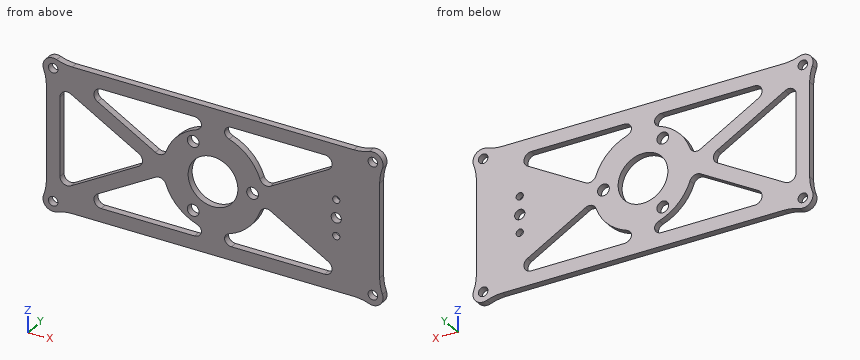
from build123d import *

# Parameters (mm, degrees)
SKETCH_1_R          = 2.1
EXTRUDE_1_DEPTH     = 3
SKETCH_1_R_2        = 22
SKETCH_1_R_3        = 2.6
SKETCH_1_R_4        = 11
EXTRUDE_1_2_DEPTH   = 3
EXTRUDE_START       = -3
EXTRUDE_2_DEPTH     = 3
FILLET_1_R          = 3.2
FILLET_2_R          = 20
EXTRUDE_4_DEPTH     = 3
SKETCH_4_R          = 2.25
SKETCH_4_R_2        = 1.6
CUT_EXTRUDE_1_DEPTH = 83.47010732


with BuildPart() as part:
    # Sketch 1 → Extrude 1 (new body)
    with BuildSketch(Plane(origin=(0, 0, 0), x_dir=(1, 0, 0), z_dir=(0, 1, 0))):
        with BuildLine():
            Line((-67.322682271, -32.275282576), (67.322682271, -32.275282576))
            ThreePointArc((67.322682271, -32.275282576), (73.858764752, -32.457263091), (73.676784237, -25.92118061))
            Line((73.676784237, -25.92118061), (73.676784237, 25.92118061))
            ThreePointArc((73.676784237, 25.92118061), (73.858764752, 32.457263091), (67.322682271, 32.275282576))
            Line((67.322682271, 32.275282576), (-67.322682271, 32.275282576))
            ThreePointArc((-67.322682271, 32.275282576), (-73.858764752, 32.457263091), (-73.676784237, 25.92118061))
            Line((-73.676784237, 25.92118061), (-73.676784237, -25.92118061))
            ThreePointArc((-73.676784237, -25.92118061), (-73.858764752, -32.457263091), (-67.322682271, -32.275282576))
        make_face()
        with Locations(Location((70.676784237, -29.275282576, 0), (0, 0, 270))):
            Circle(SKETCH_1_R, mode=Mode.SUBTRACT)
        with Locations(Location((-70.676784237, -29.275282576, 0), (0, 0, 270))):
            Circle(SKETCH_1_R, mode=Mode.SUBTRACT)
        with Locations(Location((70.676784237, 29.275282576, 0), (0, 0, 270))):
            Circle(SKETCH_1_R, mode=Mode.SUBTRACT)
        with Locations(Location((-70.676784237, 29.275282576, 0), (0, 0, 270))):
            Circle(SKETCH_1_R, mode=Mode.SUBTRACT)
        with BuildLine():
            Line((-67.322682271, 26.275282576), (67.322682271, 26.275282576))
            ThreePointArc((67.322682271, 26.275282576), (67.494803722, 26.093302061), (67.676784237, 25.92118061))
            Line((67.676784237, 25.92118061), (67.676784237, -25.92118061))
            ThreePointArc((67.676784237, -25.92118061), (67.494803722, -26.093302061), (67.322682271, -26.275282576))
            Line((67.322682271, -26.275282576), (-67.322682271, -26.275282576))
            ThreePointArc((-67.322682271, -26.275282576), (-67.494803722, -26.093302061), (-67.676784237, -25.92118061))
            Line((-67.676784237, -25.92118061), (-67.676784237, 25.92118061))
            ThreePointArc((-67.676784237, 25.92118061), (-67.494803722, 26.093302061), (-67.322682271, 26.275282576))
        make_face(mode=Mode.SUBTRACT)
    extrude(amount=EXTRUDE_1_DEPTH)



with BuildPart() as body_2:
    # Sketch 1 → Extrude 1 2 (new body)
    with BuildSketch(Plane(origin=(0, 0, 0), x_dir=(1, 0, 0), z_dir=(0, 1, 0))):
        with Locations(Location((0, 0, 0), (0, 0, 270))):
            Circle(SKETCH_1_R_2)
        with Locations(Location((-8.75, 15.155444566, 0), (0, 0, 270))):
            Circle(SKETCH_1_R_3, mode=Mode.SUBTRACT)
        with Locations(Location((0, 0, 0), (0, 0, 270))):
            Circle(SKETCH_1_R_4, mode=Mode.SUBTRACT)
        with Locations(Location((-8.75, -15.155444566, 0), (0, 0, 270))):
            Circle(SKETCH_1_R_3, mode=Mode.SUBTRACT)
        with Locations(Location((17.5, 0, 0), (0, 0, 270))):
            Circle(SKETCH_1_R_3, mode=Mode.SUBTRACT)
    extrude(amount=EXTRUDE_1_2_DEPTH)


with BuildPart() as part_1:
    add(part.part)

    add(body_2.part)  # Extrude 2 merges body 2
    # Sketch 2 → Extrude 2 (add)
    with BuildSketch(Plane(origin=(0, 3, 0), x_dir=(1, 0, 0), z_dir=(0, 1, 0)).offset(EXTRUDE_START)):
        with BuildLine():
            Line((-5, 26.275282576), (-5, 21.424285286))
            ThreePointArc((-5, 21.424285286), (0, 22), (5, 21.424285286))
            Line((5, 21.424285286), (5, 26.275282576))
            Line((5, 26.275282576), (-5, 26.275282576))
        make_face()
        with BuildLine():
            Line((5, -26.275282576), (5, -21.424285286))
            ThreePointArc((5, -21.424285286), (0, -22), (-5, -21.424285286))
            Line((-5, -21.424285286), (-5, -26.275282576))
            Line((-5, -26.275282576), (5, -26.275282576))
        make_face()
        with BuildLine():
            Line((-67.676784237, 23.012880146), (-27.981475463, 0))
            Line((-27.981475463, 0), (-67.676784237, -23.012880146))
            Line((-67.676784237, -23.012880146), (-67.676784237, -25.92118061))
            ThreePointArc((-67.676784237, -25.92118061), (-67.494803722, -26.093302061), (-67.322682271, -26.275282576))
            Line((-67.322682271, -26.275282576), (-61.341206808, -26.275282576))
            Line((-61.341206808, -26.275282576), (-21.747820556, -3.321490792))
            ThreePointArc((-21.747820556, -3.321490792), (-22, 0), (-21.747820556, 3.321490792))
            Line((-21.747820556, 3.321490792), (-61.341206808, 26.275282576))
            Line((-61.341206808, 26.275282576), (-67.322682271, 26.275282576))
            ThreePointArc((-67.322682271, 26.275282576), (-67.494803722, 26.093302061), (-67.676784237, 25.92118061))
            Line((-67.676784237, 25.92118061), (-67.676784237, 23.012880146))
        make_face()
        with BuildLine():
            Line((61.341206808, 26.275282576), (21.747820556, 3.321490792))
            ThreePointArc((21.747820556, 3.321490792), (22, 0), (21.747820556, -3.321490792))
            Line((21.747820556, -3.321490792), (61.341206808, -26.275282576))
            Line((61.341206808, -26.275282576), (67.322682271, -26.275282576))
            ThreePointArc((67.322682271, -26.275282576), (67.494803722, -26.093302061), (67.676784237, -25.92118061))
            Line((67.676784237, -25.92118061), (67.676784237, -23.012880146))
            Line((67.676784237, -23.012880146), (27.981475463, 0))
            Line((27.981475463, 0), (67.676784237, 23.012880146))
            Line((67.676784237, 23.012880146), (67.676784237, 25.92118061))
            ThreePointArc((67.676784237, 25.92118061), (67.494803722, 26.093302061), (67.322682271, 26.275282576))
            Line((67.322682271, 26.275282576), (61.341206808, 26.275282576))
        make_face()
    extrude(amount=EXTRUDE_2_DEPTH)

    # Fillet 1
    # the kernel refuses this fillet: 3.2 mm, written as the material it adds along each edge
    with BuildSketch(Plane(origin=(-27.981475463, 0, 0), x_dir=(-0.8651295335829952, 0, -0.5015484922940843), z_dir=(0, 1, 0))) as fillet_1_piece_1:
        with BuildLine():
            CenterArc((FILLET_1_R * 1.72491702572, FILLET_1_R), FILLET_1_R, 150.205000829, 119.794999171)
            Line((FILLET_1_R * 0.857108199306, FILLET_1_R * 1.49689821976), (0, 0))
            Line((0, 0), (FILLET_1_R * 1.72491702572, 0))
        make_face()
    extrude(amount=3)
    with BuildSketch(Plane(origin=(-67.676784237, 0, 23.012880146), x_dir=(0, 0, -1), z_dir=(0, 1, 0))) as fillet_1_piece_2:
        with BuildLine():
            CenterArc((FILLET_1_R * 1.73563429984, -FILLET_1_R), FILLET_1_R, 90, 120.102500415)
            Line((FILLET_1_R * 0.87050476626, -FILLET_1_R * 1.50154849229), (0, 0))
            Line((0, 0), (FILLET_1_R * 1.73563429984, 0))
        make_face()
    extrude(amount=3)
    with BuildSketch(Plane(origin=(5, 0, 21.424285286), x_dir=(0, 0, 1), z_dir=(0, 1, 0)), Plane(origin=(-5, 0, -21.424285286), x_dir=(0, 0, -1), z_dir=(0, 1, 0))) as fillet_1_piece_3:
        with BuildLine():
            CenterArc((2.404269014, 3.2), FILLET_1_R, 198.989618262, 71.010381738)
            ThreePointArc((-0.621579151, 2.158730159), (-0.283217903, 1.087303995), (0, 0))
            Line((0, 0), (2.404269014, 0))
        make_face()
    extrude(amount=3)
    with BuildSketch(Plane(origin=(21.747820556, 0, 3.321490792), x_dir=(0.8651295335829955, 0, 0.5015484922940839), z_dir=(0, 1, 0)), Plane(origin=(-21.747820556, 0, -3.321490792), x_dir=(-0.8651295335829956, 0, -0.5015484922940837), z_dir=(0, 1, 0))) as fillet_1_piece_4:
        with BuildLine():
            CenterArc((4.251428919, -3.2), FILLET_1_R, 90, 101.059486295)
            ThreePointArc((1.110857558, -3.813849756), (0.641683834, -1.881801424), (0, 0))
            Line((0, 0), (4.251428919, 0))
        make_face()
    extrude(amount=3)
    with BuildSketch(Plane(origin=(61.341206808, 0, 26.275282576), x_dir=(-0.8651295335829955, 0, -0.5015484922940838), z_dir=(0, 1, 0)), Plane(origin=(61.341206808, 0, -26.275282576), x_dir=(-1, 0, 0), z_dir=(0, 1, 0)), Plane(origin=(-61.341206808, 0, 26.275282576), x_dir=(1, 0, 0), z_dir=(0, 1, 0))) as fillet_1_piece_5:
        with BuildLine():
            CenterArc((FILLET_1_R * 3.71874217995, FILLET_1_R), FILLET_1_R, 120.102500415, 149.897499585)
            Line((FILLET_1_R * 3.21719368765, FILLET_1_R * 1.86512953358), (0, 0))
            Line((0, 0), (FILLET_1_R * 3.71874217995, 0))
        make_face()
    extrude(amount=3)
    with BuildSketch(Plane(origin=(5, 0, 26.275282576), x_dir=(1, 0, 0), z_dir=(0, 1, 0)), Plane(origin=(-5, 0, -26.275282576), x_dir=(-1, 0, 0), z_dir=(0, 1, 0)), Plane(origin=(5, 0, -26.275282576), x_dir=(0, 0, 1), z_dir=(0, 1, 0)), Plane(origin=(-5, 0, 26.275282576), x_dir=(0, 0, -1), z_dir=(0, 1, 0))) as fillet_1_piece_6:
        with BuildLine():
            CenterArc((FILLET_1_R, FILLET_1_R), FILLET_1_R, 180, 90)
            Line((0, FILLET_1_R), (0, 0))
            Line((0, 0), (FILLET_1_R, 0))
        make_face()
    extrude(amount=3)
    with BuildSketch(Plane(origin=(-61.341206808, 0, -26.275282576), x_dir=(1, 0, 0), z_dir=(0, 1, 0))) as fillet_1_piece_7:
        with BuildLine():
            CenterArc((FILLET_1_R * 3.71874217995, -FILLET_1_R), FILLET_1_R, 90, 149.897499585)
            Line((FILLET_1_R * 3.21719368765, -FILLET_1_R * 1.86512953358), (0, 0))
            Line((0, 0), (FILLET_1_R * 3.71874217995, 0))
        make_face()
    extrude(amount=3)
    with BuildSketch(Plane(origin=(21.747820556, 0, -3.321490792), x_dir=(0.8651295335829948, 0, -0.5015484922940848), z_dir=(0, 1, 0)), Plane(origin=(-21.747820556, 0, 3.321490792), x_dir=(-0.8651295335829947, 0, 0.5015484922940853), z_dir=(0, 1, 0))) as fillet_1_piece_8:
        with BuildLine():
            CenterArc((4.251428919, 3.2), FILLET_1_R, 168.940513705, 101.059486295)
            ThreePointArc((1.110857558, 3.813849756), (0.641683834, 1.881801424), (0, 0))
            Line((0, 0), (4.251428919, 0))
        make_face()
    extrude(amount=3)
    with BuildSketch(Plane(origin=(5, 0, -21.424285286), x_dir=(0, 0, -1), z_dir=(0, 1, 0)), Plane(origin=(-5, 0, 21.424285286), x_dir=(0, 0, 1), z_dir=(0, 1, 0))) as fillet_1_piece_9:
        with BuildLine():
            CenterArc((2.404269014, -3.2), FILLET_1_R, 90, 71.010381738)
            ThreePointArc((-0.621579151, -2.158730159), (-0.283217903, -1.087303995), (0, 0))
            Line((0, 0), (2.404269014, 0))
        make_face()
    extrude(amount=3)
    with BuildSketch(Plane(origin=(-67.676784237, 0, -23.012880146), x_dir=(0, 0, 1), z_dir=(0, 1, 0))) as fillet_1_piece_10:
        with BuildLine():
            CenterArc((FILLET_1_R * 1.73563429984, FILLET_1_R), FILLET_1_R, 149.897499585, 120.102500415)
            Line((FILLET_1_R * 0.87050476626, FILLET_1_R * 1.50154849229), (0, 0))
            Line((0, 0), (FILLET_1_R * 1.73563429984, 0))
        make_face()
    extrude(amount=3)

    # Fillet 2
    fillet_2_edges = [part_1.edges().sort_by_distance(p)[0] for p in [
        (-67.322682271, 1.5, 32.275282576),
        (-73.676784237, 1.5, 25.92118061),
        (-73.676784237, 1.5, -25.92118061),
        (-67.322682271, 1.5, -32.275282576),
        (67.322682271, 1.5, -32.275282576),
        (73.676784237, 1.5, -25.92118061),
        (73.676784237, 1.5, 25.92118061),
        (67.322682271, 1.5, 32.275282576),
    ]]
    fillet(fillet_2_edges, radius=FILLET_2_R)

    # Sketch 3 → Extrude 4 (add)
    with BuildSketch(Plane(origin=(0, 3, 0), x_dir=(1, 0, 0), z_dir=(0, 1, 0))):
        Polygon((67.676784237, 23.012880146), (27.981475463, 0), (67.676784237, -23.012880146), align=None)
    extrude(amount=-EXTRUDE_4_DEPTH)

    # Sketch 4 → Cut-Extrude 1 (cut, through all)
    with BuildSketch(Plane(origin=(0, 3, 0), x_dir=(1, 0, 0), z_dir=(0, 1, 0))):
        with Locations(Location((54.5, 0, 0), (0, 0, 270))):
            Circle(SKETCH_4_R)
        with Locations(Location((54.5, 8, 0), (0, 0, 270))):
            Circle(SKETCH_4_R_2)
        with Locations(Location((54.5, -8, 0), (0, 0, 270))):
            Circle(SKETCH_4_R_2)
    extrude(amount=-CUT_EXTRUDE_1_DEPTH, mode=Mode.SUBTRACT)


solid = part_1.part
Build history of the part. All positions in model axes, mm. Round coordinates to 2 decimals unless told otherwise and drop trailing zeros. Loops run counter-clockwise (first coordinate to the right, second up) from the corner with the lowest first, then second, coordinate; pieces in that order, holes last. Notation, with made-up numbers: (-19.5, -22.5) -> (28.5, -22.5) arc R29 cw to (28.5, 16.5) -> close; hole circle Ø9 at (10.25, 31). An arc over 180 degrees is marked (long way). Answer in a Markdown table with one row per item.
Item 1: Drill centre lines: L1, parallel to X at y = 2.4, z = 19.5; L2, parallel to Z at x = 8.5, y = 2.6; L3, parallel to X at y = 1.1, z = -16. Where is each one in solid material? Low to high. Write a range as [from, to].
Answers below:
| item | result |
|---|---|
| L1 | x = [-73.68, -66.94], [-61.62, -49.65], [-10.19, 10.19], [49.65, 73.68] |
| L2 | z = [-32.28, -26.28], [-20.29, -6.98], [6.98, 20.29], [26.28, 32.28] |
| L3 | x = [-73.68, -67.68], [-55.58, -43.62], [-15.1, -11.21], [-6.29, 15.1], [43.62, 73.68] |
Item 2: Saw through at D-D (y = 0.7). State how many separate pieces and enclosed holes the cut face has, and give its area (3 significant figures).
Answers below:
| item | result |
|---|---|
| separate pieces | 1 |
| enclosed holes | 16 |
| area | 5,790 mm² |
Item 3: Pin check, flat tips, straight feed: pin 1 (0.9 mm diameter, centred on x = -32, y = 2, fed in from +Z); pin 2 (0.9 mm diameter, centred on x = -22, y = 2, fed in from -Z); pin 3 (1.5 mm diameter, centred on y = 1.5, z = 3.5, fed in from +X). Stop position of each tip, or through.
Answers below:
| item | result |
|---|---|
| pin 1 | stops at z = 32.28 |
| pin 2 | stops at z = -32.28 |
| pin 3 | stops at x = 73.68 |
Item 4: Saw through at C-C (x = 54.5). Write the cut outline in (y, z), and give its area (3 significant figures).
Answers below:
| item | result |
|---|---|
| outline | (0, -32.28) -> (3, -32.28) -> (3, -9.6) -> (0, -9.6) -> close; (0, -6.4) -> (3, -6.4) -> (3, -2.25) -> (0, -2.25) -> close; (0, 2.25) -> (3, 2.25) -> (3, 6.4) -> (0, 6.4) -> close; (0, 9.6) -> (3, 9.6) -> (3, 32.28) -> (0, 32.28) -> close |
| area | 161 mm² |
Item 5: Saw through at A-A (z = 0). Write the cut outline in (x, y).
Answers below:
| item | result |
|---|---|
| outline | (-73.68, 0) -> (-67.68, 0) -> (-67.68, 3) -> (-73.68, 3) -> close; (-31.16, 0) -> (-11, 0) -> (-11, 3) -> (-31.16, 3) -> close; (11, 0) -> (14.9, 0) -> (14.9, 3) -> (11, 3) -> close; (20.1, 0) -> (52.25, 0) -> (52.25, 3) -> (20.1, 3) -> close; (56.75, 0) -> (73.68, 0) -> (73.68, 3) -> (56.75, 3) -> close |
Item 6: Saw through at B-B (x = 0). Write the cut outline in (y, z).
Answers below:
| item | result |
|---|---|
| outline | (0, -32.28) -> (3, -32.28) -> (3, -11) -> (0, -11) -> close; (0, 11) -> (3, 11) -> (3, 32.28) -> (0, 32.28) -> close |
